from build123d import *

# Parameters (mm, degrees)
F1_DEPTH = 63.5
F2_DEPTH = 25.4
F3_DEPTH = 7.9375
F0_W     = 32.035574
F0_H     = 28.575
F5_R     = 6.35


with BuildPart() as f1:
    # F0 (on Front) → F1 (new body, symmetric)
    with BuildSketch(Plane.XZ):
        Polygon((-41.275, 9.525), (-41.275, -9.525), (41.275, -9.525), (41.275, 9.525), (22.225, 9.525), align=None)
    extrude(amount=F1_DEPTH, both=True)

    # F0 (on Front) → F2 (join, symmetric)
    with BuildSketch(Plane.XZ):
        with BuildLine():
            Line((22.225, 9.525), (41.275, 9.525))
            Line((41.275, 9.525), (41.275, 27.0002))
            ThreePointArc((41.275, 27.0002), (45.92468, 38.22552), (57.15, 42.8752))
            Line((57.15, 42.8752), (60.325, 42.8752))
            Line((60.325, 42.8752), (60.325, 61.9252))
            Line((60.325, 61.9252), (57.15, 61.9252))
            add(Edge.make_bspline(
                [(56.676857, 61.921995), (56.834796, 61.923482), (56.992512, 61.924551), (57.15, 61.9252)],
                knots=[111.078345, 111.078345, 111.078345, 111.078345, 111.504536, 111.504536, 111.504536, 111.504536], degree=3))
            ThreePointArc((56.676857, 61.921995), (32.287577, 51.528053), (22.225, 27.0002))
            Line((22.225, 27.0002), (22.225, 9.525))
        make_face()
    extrude(amount=F2_DEPTH, both=True)

    # F0 (on Front) → F3 (join, symmetric)
    with BuildSketch(Plane.XZ):
        with BuildLine():
            add(Edge.make_bspline(
                [(-41.275, 9.525), (-40.855104, 32.748828), (15.513022, 61.534422), (56.676857, 61.921995)],
                knots=[0, 0, 0, 0, 111.078345, 111.078345, 111.078345, 111.078345], degree=3))
            Line((-41.275, 9.525), (22.225, 9.525))
            Line((22.225, 9.525), (22.225, 27.0002))
            ThreePointArc((22.225, 27.0002), (32.287577, 51.528053), (56.676857, 61.921995))
        make_face()
    extrude(amount=F3_DEPTH, both=True)

    # F0 (on Front) → F4 (revolve)
    with BuildSketch(Plane.XZ):
        with Locations((95.107213, 52.3875)):
            Rectangle(F0_W, F0_H)
    revolve(axis=Axis((79.089426, 0, 52.3875), (0, 0, 1)))

    # F5
    f5_edges = [f1.edges().sort_by_distance(p)[0] for p in [
        (41.275, -63.5, 0),
        (-41.275, -63.5, 0),
        (41.275, 63.5, 0),
        (-41.275, 63.5, 0),
    ]]
    fillet(f5_edges, radius=F5_R)


solid = f1.part
Verification items for the finished model (mm, model axes). A direction names the side the tool comes from. Round coordinates to 2 decimals unless told otherwise and drop trailing zeros. Loops run counter-clockwise (first coordinate to the right, second up) from the corner with the lowest first, then second, coordinate; pieces in that order, holes last. Notation, with made-up numbers: (65.25, 85) - (70.25, 85) arc R18 ccw to (70.25, 114) - close; hole circle Ø10 at (0.25, 84.25). An arc over 180 degrees is marked (long way). Answer in a Markdown table with one row per item. Add a question column.
Q1. Release check for a two-part mould opening along X. For faces 4 (the face through (36, -25.4, 36)), 5 (the face through (39.464, -61.59, 0.133)), 6 (the face through (44.047, -0.356, 35.962)) record: pulls with the +X half, pulls with the -X half, needs draft (parallel to the pull), parting line crosses it, or undercut.
Q2. Section check A-A on y = -40. Enter the section's corners in (x, z) (3 decimals), plus the area to 3 significant figures.
Q3. Section check C-C on y = -10.5. Enter the section's corners in (x, z) (3 decimals), plus the area to 3 significant figures.
Q4. Material ranges on line 1 (Y direction, x = 5.5, z = 16); line 2 (X direction, y = 51, z = -2) (3 decimals); line 3 (Y direction, x = 54, z = 55), recorded low to high.
Q5. Tool access check on faces 1 (the face through (41.275, -1, 4)), 2 (the face through (32.56, -16.79, 51.8)), 3 (the face through (36, 25.4, 36)). Record the directions out of +Z, -Z, +X, -X, +Y, -Y that give a thin tool (end or side, any length) a straight path to the whole face; none if there is none.
Q6. Section check B-B on x = 64. Enter the section's corners in (y, z) (3 decimals).
Q7. Gauge pin test, flat ends, axial feed: pin 1 (1 mm diameter, centred on x = 58, y = 24.5, fed in from -Z); pin 2 (18.5 mm diameter, centred on x = 47.5, z = 24, fed in from +Y); pin 3 (4 mm diameter, centred on y = 39, z = 13, fed in from -X); pin 4 (10 mm diameter, centred on x = 44, z = 9.5, fed in from +Y). Record the tip position at first contact, or that the pin passes through.
Found:
| question | item | result |
|---|---|---|
| 1 | face 4 | needs draft |
| 1 | face 5 | pulls with the +X half |
| 1 | face 6 | undercut |
| 2 | outline | (-41.275, -9.525) - (41.275, -9.525) - (41.275, 9.525) - (-41.275, 9.525) - close |
| 2 | area | 1,570 mm² |
| 3 | outline | (-41.275, -9.525) - (41.275, -9.525) - (41.275, 27) arc R15.875 cw to (48.823, 40.516) - (48.823, 38.1) - (109.355, 38.1) - (109.355, 66.675) - (48.823, 66.675) - (48.823, 60.918) arc R34.925 ccw to (22.225, 27) - (22.225, 9.525) - (-41.275, 9.525) - close |
| 3 | area | 4,230 mm² |
| 4 | line 1 | y = -7.94 to 7.94 |
| 4 | line 2 | x = -41.275 to 41.275 |
| 4 | line 3 | y = -25.4 to 25.4 |
| 5 | face 1 | -Z, +X, +Y, -Y |
| 5 | face 2 | +Z, -X, -Y |
| 5 | face 3 | +Z, -X, +Y |
| 6 | outline | (-28.259, 38.1) - (28.259, 38.1) - (28.259, 66.675) - (-28.259, 66.675) - close |
| 7 | pin 1 | stops at z = 38.1 |
| 7 | pin 2 | stops at y = 25.4 |
| 7 | pin 3 | passes through |
| 7 | pin 4 | stops at y = 62.02 |
